Model file for the job. Use its own axes, mm. A direction names the side the tool comes from. Give positions to 0.01 mm unless a question says otherwise; leave off trailing zeros. Write each loop counter-clockwise with the first axis right and the second up, starting at its lowest first coordinate (ties: lowest second). Pieces come first, ordered by that corner, then holes.
```python
from build123d import *

# Parameters (mm, degrees)
SKETCH1_R               = 30.35
BOSS_EXTRUDE1_DEPTH     = 10
SKETCH2_R               = 30.35
BOSS_EXTRUDE2_DEPTH     = 140.65
SKETCH4_R               = 25.35
CUT_EXTRUDE1_DEPTH      = 308.65
SKETCH6_R               = 2.55
CUT_EXTRUDE3_DEPTH      = 90
CUT_EXTRUDE4_START      = -6
CUT_EXTRUDE4_DEPTH      = 7
CUT_EXTRUDE5_DEPTH      = 10
CUT_EXTRUDE6_DEPTH      = 137
CUT_EXTRUDE6_DEPTH_BACK = 137
SKETCH10_R              = 4.05


with BuildPart() as part:
    # Sketch1 → Boss-Extrude1 (new body)
    with BuildSketch(Plane(origin=(0, 0, 0), x_dir=(1, 0, 0), z_dir=(0, 1, 0))):
        with Locations(Location((0, 0, 0), (0, 0, 270))):
            Circle(SKETCH1_R)
    extrude(amount=BOSS_EXTRUDE1_DEPTH)

    # Sketch2 → Boss-Extrude2 (add)
    with BuildSketch(Plane(origin=(0, 10, 0), x_dir=(1, 0, 0), z_dir=(0, 1, 0))):
        with Locations(Location((0, 0, 0), (0, 0, 270))):
            Circle(SKETCH2_R)
    extrude(amount=BOSS_EXTRUDE2_DEPTH)

    # Sketch4 → Cut-Extrude1 (cut)
    with BuildSketch(Plane(origin=(0, 150.65, 0), x_dir=(1, 0, 0), z_dir=(0, 1, 0))):
        with Locations(Location((0, 0, 0), (0, 0, 270))):
            Circle(SKETCH4_R)
    extrude(amount=-CUT_EXTRUDE1_DEPTH, mode=Mode.SUBTRACT)

    # Sketch6 → Cut-Extrude3 (cut)
    with BuildSketch(Plane(origin=(0, 0, -30.35), x_dir=(-1, 0, 0), z_dir=(0, 0, -1))):
        with Locations((0, 5)):
            Circle(SKETCH6_R)
    extrude(amount=-CUT_EXTRUDE3_DEPTH, mode=Mode.SUBTRACT)

    # Cut-Extrude4: read off the stored shape, not the designer's step
    # Cut-Extrude4 outline → Cut-Extrude4 (cut)
    with BuildSketch(Plane(origin=(-21.460690809, 0, -21.460690809), x_dir=(0, -1, 0), z_dir=(-0.7071067811865417, 0, -0.7071067811865533)).offset(CUT_EXTRUDE4_START)):
        with BuildLine():
            ThreePointArc((-106.74, 2.55), (-109.29, 0), (-106.74, -2.55))
            Line((-106.74, -2.55), (-86.74, -2.55))
            ThreePointArc((-86.74, -2.55), (-84.19, 0), (-86.74, 2.55))
            Line((-86.74, 2.55), (-106.74, 2.55))
        make_face()
    extrude(amount=CUT_EXTRUDE4_DEPTH, mode=Mode.SUBTRACT)

    # Sketch9 → Cut-Extrude5 (cut)
    with BuildSketch(Plane(origin=(-21.460690809, 0, 21.460690809), x_dir=(0, -1, 0), z_dir=(-0.7071067811865512, 0, 0.7071067811865438))):
        with BuildLine():
            Line((-86.74, 2.55), (-106.74, 2.55))
            ThreePointArc((-106.74, 2.55), (-109.29, 0), (-106.74, -2.55))
            Line((-106.74, -2.55), (-86.74, -2.55))
            ThreePointArc((-86.74, -2.55), (-84.19, 0), (-86.74, 2.55))
        make_face()
    extrude(amount=-CUT_EXTRUDE5_DEPTH, mode=Mode.SUBTRACT)

    # Sketch10 → Cut-Extrude6 (cut, two sides: drawn at the far end of the back side and taken through both)
    with BuildSketch(Plane(origin=(0, 0, 0), x_dir=(0, 0, -1), z_dir=(1, 0, 0)).offset(-CUT_EXTRUDE6_DEPTH_BACK)):
        with Locations(Location((0, 130.65, 0), (0, 0, 180))):
            Circle(SKETCH10_R)
    extrude(amount=CUT_EXTRUDE6_DEPTH + CUT_EXTRUDE6_DEPTH_BACK, mode=Mode.SUBTRACT)


solid = part.part
```
1. Slice it at C-C, the plane y = 130.65. Write the cut outline in (x, z).
Calculated:
outline: (-30.08, -4.05) arc R30.35 ccw to (30.08, -4.05) - (25.02, -4.05) arc R25.35 cw to (-25.02, -4.05) - close; (-30.08, 4.05) - (-25.02, 4.05) arc R25.35 cw to (25.02, 4.05) - (30.08, 4.05) arc R30.35 ccw to start
2. Slice it at B-B, the plane z = 0. Write the cut outline in (x, y), and give its area (3 significant figures).
Calculated:
outline: (-30.35, 0) - (-25.35, 0) - (-25.35, 126.6) - (-30.35, 126.6) - close; (-30.35, 134.7) - (-25.35, 134.7) - (-25.35, 150.65) - (-30.35, 150.65) - close; (25.35, 0) - (30.35, 0) - (30.35, 126.6) - (25.35, 126.6) - close; (25.35, 134.7) - (30.35, 134.7) - (30.35, 150.65) - (25.35, 150.65) - close
area: 1,430 mm2
3. Slice it at A-A, the plane x = 0. Write the cut outline in (y, z), and give its area (3 significant figures).
Calculated:
outline: (0, -30.35) - (2.45, -30.35) - (2.45, -25.35) - (0, -25.35) - close; (0, 25.35) - (2.45, 25.35) - (2.45, 30.35) - (0, 30.35) - close; (7.55, -30.35) - (150.65, -30.35) - (150.65, -25.35) - (7.55, -25.35) - close; (7.55, 25.35) - (150.65, 25.35) - (150.65, 30.35) - (7.55, 30.35) - close
area: 1,460 mm2
4. Pull direction Z, two halves, no side cores. Call faces 1 (the cylindrical face through (30.09, 74.27, -3.95)), 2 (the flat face through (-25, 150.65, -7)), 3 (the cylindrical face through (-19.58, 84.19, -19.66)): +Z half, -Z half, draft (parallel to the pull), parting line (faces both ways), or undercut.
Calculated:
face 1: parting line
face 2: draft
face 3: undercut
5. Which spindle directions (+Z, -Z, +X, -X, +Y, -Y) get a long thin tool onto all of the face, cutting with end or side? Do faces 4 (the flat face through (-21.437, 96.88, 17.831)), 5 (the flat face through (-17.831, 96.6, 21.437)), 6 (the cylindrical face through (-19.66, 109.29, -19.58)). Say none if no direction does.
Calculated:
face 4: +Z
face 5: -X
face 6: none
6. Pin check, flat tips, straight feed: P1, Ø6, axis at x = 24.5, y = 42, coming from the +Z side; P2, Ø5, axis at y = 28.5, z = 22, coming from the -X side; P3, Ø3, axis at x = 0, y = 5, coming from the +Z side; P4, Ø4, axis at y = 62.5, z = -12.5, coming from the +X side. Stop position of each tip, or through.
Calculated:
P1: stops at z = 21.42
P2: stops at x = -23.26
P3: passes through
P4: stops at x = 28.48
7. Probe probe 1 along Z at (x, y) = (0, 55); probe 2 along Y at (x, z) = (-27.7, 0); probe 3 along Y at (x, z) = (0, 28.1). List the from-to ranges inside material, lowest first.
Calculated:
probe 1: z = -30.35 to -25.35, 25.35 to 30.35
probe 2: y = 0 to 126.6, 134.7 to 150.65
probe 3: y = 0 to 2.45, 7.55 to 150.65
8. Slice it at D-D, the plane x = 23.5. Write the cut outline in (y, z).
Calculated:
outline: (0, -19.21) - (150.65, -19.21) - (150.65, -9.51) - (0, -9.51) - close; (0, 9.51) - (150.65, 9.51) - (150.65, 19.21) - (0, 19.21) - close
